The model under review builds one solid part; all positions refer to its coordinate system, in mm. A direction names the side the tool comes from. Give positions to 0.01 mm unless a question says otherwise; leave off trailing zeros. Order: outer loops, then holes, each group sorted by start corner. A loop starts at its lowest first (then second) coordinate and runs counter-clockwise, first axis right, second up. Notation, with made-up numbers: M 4.25,-23.75 L 15.25,-23.75 A21 cw 15.25,5.25 Z; hole C 0,81 d3. An arc over 180 degrees is marked long. One line per question, with ' | ' between items. Start each with the question number.
1. Wall thickness on L1, parallel to Z at x = 120, y = 117.25; L2, parallel to Y at x = 86.5, z = 4.25; L3, parallel to X at y = 118.75, z = 15: over which ranges is each line inside the solid? List them lowest first.
2. We need section C-C on z = 16. Write out the cut boundary in (x, y).
3. For faces 1 (the face through (100, 124, 28.5)), 2 (the face through (125, 124, 15)), list the 3-axis set-ups (+Z, -Z, +X, -X, +Y, -Y) from which the entire face can be reached by the end or side of a thin tool; tool diameter is ignored.
4. We need section A-A on y = 121. Write out the cut boundary in (x, z).
5. We need section B-B on x = 81. Write out the cut boundary in (y, z), then the cut area to 3 significant figures.
6. Insertion check: P1, Ø5, axis at y = 123, z = 14.5, coming from the -X side; P2, Ø8, axis at x = 87, y = 128.5, coming from the -Z side. Each pin has a flat end and moves straight along its axis. Give the tip position at first contact, or say it passes through.
7. The part is to be moulded in two halves that separate along Z. For faces 3 (the face through (77.5, 132, 15)), 4 (the face through (100, 131.4, 15)), 5 (the face through (101, 124, 30)), say which applies: +Z half, -Z half, draft (parallel to the pull), parting line (faces both ways), or undercut.
```python
from build123d import *

# Parameters (mm, degrees)
BOX026_W     = 47.5
BOX026_H     = 16
BOX026_DEPTH = 27
BOX027_W     = 47.5
BOX027_H     = 17.5
BOX027_DEPTH = 30


with BuildPart() as cube026:
    # Box026 → Box026 (new body)
    with BuildSketch(Plane(origin=(-1.5, 0, 60), x_dir=(1, 0, 0), z_dir=(0, 0, 1))):
        with Locations((23.75, 8)):
            Rectangle(BOX026_W, BOX026_H)
    extrude(amount=BOX026_DEPTH)


with BuildPart() as cut035:
    # Box027 → Box027 (new body)
    with BuildSketch(Plane.XY.offset(58.5)):
        with Locations((23.75, 8.75)):
            Rectangle(BOX027_W, BOX027_H)
    extrude(amount=BOX027_DEPTH)

    # Cut035: cut Cube026
    add(cube026.part, mode=Mode.SUBTRACT)


with BuildPart() as cut035_1:
    # Cut035 placement: moved
    add(cut035.part.moved(Location((77.5, 115.4, -58.5))))


solid = cut035_1.part
```
Entries:
1) L1: z = 0 to 1.5, 28.5 to 30 | L2: y = 131.4 to 132.9 | L3: x = 123.5 to 125
2) outline: M 77.5,131.4 L 123.5,131.4 L 123.5,115.4 L 125,115.4 L 125,132.9 L 77.5,132.9 Z
3) face 1: -X, -Y | face 2: +Z, -Z, +X, +Y, -Y
4) outline: M 77.5,0 L 125,0 L 125,30 L 77.5,30 L 77.5,28.5 L 123.5,28.5 L 123.5,1.5 L 77.5,1.5 Z
5) outline: M 115.4,0 L 132.9,0 L 132.9,30 L 115.4,30 L 115.4,28.5 L 131.4,28.5 L 131.4,1.5 L 115.4,1.5 Z | area: 93.0 mm^2
6) P1: stops at x = 123.5 | P2: stops at z = 0
7) face 3: draft | face 4: undercut | face 5: +Z half
